Autodesk Inventor part; units mm, degrees
ref_plane "YZ Plane" through (0, 0, 0) normal (1, 0, 0) x (0, 1, 0)
ref_plane "XZ Plane" through (0, 0, 0) normal (0, 1, 0) x (-1, 0, 0)
ref_plane "XY Plane" through (0, 0, 0) normal (0, 0, 1) x (1, 0, 0)
sketch "Boceto1" plane through (0, 0, 0) normal (0, 0, 1) x (1, 0, 0)
  circle A0 centre (0, 0) radius 10
  dimension "d0" = 20
extrude "Extrusión1" add sketch "Boceto1" along normal blind 110
sketch "Boceto2" plane through (0, 0, 110) normal (0, 0, 1) x (1, 0, 0)
  line L0 (2.5, -6) -> (-2.5, -6)
  line L1 (-2.5, -6) -> (-2.5, 6)
  line L2 (-2.5, 6) -> (2.5, 6)
  line L3 (2.5, 6) -> (2.5, -6)
  line L4 (2.5, -6) -> (-2.5, 6) construction
  line L5 (-2.5, -6) -> (2.5, 6) construction
  point P0 (0, 0)
  dimension "d3" = 5
  dimension "d4" = 12
extrude "Extrusión2" add sketch "Boceto2" along normal blind 30
sketch "Boceto3" plane through (-2.5, -6, 110) normal (-1, 0, 0) x (0, 0, 1)
  circle A0 centre (24, 6) radius 4
  line L0 (30, 12) -> (30, 0)
  line L1 (0, 12) -> (30, 12)
  point P0 (-110, 6)
  dimension "d7" = 8
  dimension "d8" = 6
  dimension "d9" = 6
extrude "Extrusión3" cut sketch "Boceto3" against normal blind 30
properties part number "cil_sierra"
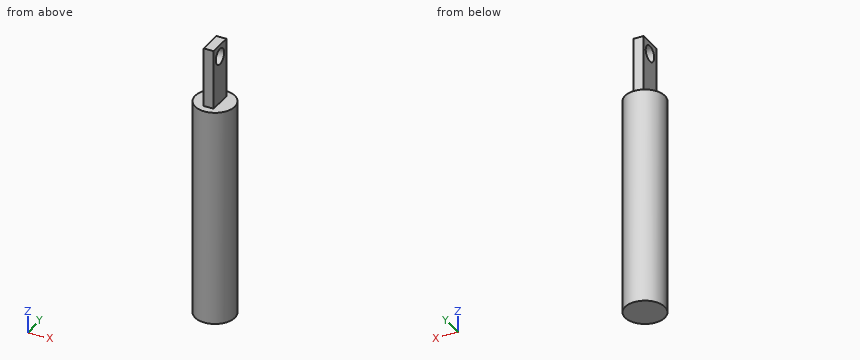
The model under review builds one solid part; all positions refer to its coordinate system, in mm. Round coordinates to 2 decimals unless told otherwise and drop trailing zeros. Loops run counter-clockwise (first coordinate to the right, second up) from the corner with the lowest first, then second, coordinate; pieces in that order, holes last. Notation, with made-up numbers: (8.5, 5) -> (22.5, 5) arc R19 cw to (22.5, 22) -> close; hole circle Ø9 at (51, -38). An arc over 180 degrees is marked (long way). Return JSON: item names as keys, results as strings.
(1) Add section A-A on y = 0. Write out the cut boundary in (x, z), plus the area to 3 significant figures.
Solved:
{"outline": "(-10, 0) -> (10, 0) -> (10, 110) -> (2.5, 110) -> (2.5, 130) -> (-2.5, 130) -> (-2.5, 110) -> (-10, 110) -> close; (-2.5, 138) -> (2.5, 138) -> (2.5, 140) -> (-2.5, 140) -> close", "area": "2,310 mm2"}
(2) Add section D-D on z = 61. Write out the cut boundary in (x, y).
Solved:
{"outline": "circle Ø20 at (0, 0)"}
(3) For line 1 (Y direction, x = -1.5, z = 134); line 2 (Z direction, x = 6, y = -5.5); line 3 (X direction, y = -2.25, z = 123.5), list the stretches that pass through material, from the lowest coordinate up.
Solved:
{"line 1": "-6 to -4, 4 to 6", "line 2": "0 to 110", "line 3": "-2.5 to 2.5"}
(4) Add section C-C on z = 134. Write out the cut boundary in (x, y).
Solved:
{"outline": "(-2.5, -6) -> (2.5, -6) -> (2.5, -4) -> (-2.5, -4) -> close; (-2.5, 4) -> (2.5, 4) -> (2.5, 6) -> (-2.5, 6) -> close"}
(5) For pin 1 (9.5 mm diameter, centred on y = 2.5, z = 125, fed in from +X); pin 2 (5.5 mm diameter, centred on x = -0.5, z = 121.5, fed in from -Y); pin 3 (8 mm diameter, centred on y = 7.5, z = 77, fed in from -X), all flat-tipped, find the tip position at first contact; note any pin that passes through.
Solved:
{"pin 1": "x = 2.5", "pin 2": "y = -6", "pin 3": "x = -9.37"}
(6) Add section B-B on x = 0. Write out the cut boundary in (y, z), plus the area to 3 significant figures.
Solved:
{"outline": "(-10, 0) -> (10, 0) -> (10, 110) -> (6, 110) -> (6, 140) -> (-6, 140) -> (-6, 110) -> (-10, 110) -> close; hole circle Ø8 at (0, 134)", "area": "2,510 mm2"}
